Autodesk Inventor part; units mm, degrees
ref_plane "YZ Plane" through (0, 0, 0) normal (1, 0, 0) x (0, 1, 0)
ref_plane "XZ Plane" through (0, 0, 0) normal (0, 1, 0) x (-1, 0, 0)
ref_plane "XY Plane" through (0, 0, 0) normal (0, 0, 1) x (1, 0, 0)
sketch "スケッチ1" plane through (0, 0, 0) normal (0, 0, 1) x (1, 0, 0)
  circle A0 centre (0, 0) radius 4.25
  circle A1 centre (0, 0) radius 4.5
  circle A2 centre (0, 0) radius 5
  line L0 (0, -5) -> (0, -6)
  line L1 (0, -6) -> (8.75, -6)
  line L2 (8.75, -6) -> (-8.75, -6)
  line L3 (0, -6) -> (11.25, -6)
  line L4 (11.25, -6) -> (-11.25, -6)
  line L5 (-11.25, -6) -> (-11.25, -4)
  line L6 (-11.25, -4) -> (11.25, -4)
  line L7 (11.25, -4) -> (11.25, -6)
  circle A3 centre (0, 0) radius 6
  line L8 (-6, 0) -> (-6, -4)
  line L9 (6, 0) -> (6, -4)
  circle A4 centre (0, 0) radius 7.2111
  line L10 (0, 0) -> (0, -3)
  line L11 (0, -3) -> (0, 7.2111)
  line L12 (0, -3) -> (0.75, -3)
  line L13 (0.75, -3) -> (-0.75, -3)
  line L14 (-0.75, -3) -> (-0.75, 5.9529)
  line L15 (0.75, -3) -> (0.75, 5.9529)
  point P0 (4.4721, -4)
  point P1 (-4.4721, -4)
  point P2 (4, -6)
  point P3 (-4, -6)
  point P4 (-0.75, 4.4371)
  point P5 (0.75, 4.4371)
  dimension "d2" = 10
  dimension "d0" = 8.5
  dimension "d1" = 9
  dimension "d3" = 1
  dimension "d4" = 8.75
  dimension "d5" = 17.5
  dimension "d6" = 11.25
  dimension "d7" = 22.5
  dimension "d8" = 2
  dimension "d9" = 12
  dimension "d18" = 3
  dimension "d19" = 0.75
  dimension "d20" = 1.5
extrude "押し出し1" add sketch "スケッチ1" along normal blind 5 contours L6 A1 A0 | A0 L6 | L6 A2 A1 | L6 A3 L0 A2 | A2 L0 A3 L6 | L6 A4 L1 A3 | A3 L2 A4 L6 | L6 L7 L3 L1 A4 | A4 L2 L4 L5 L6
extrude "押し出し2" add sketch "スケッチ1" along normal blind 3 contours A0 L6 L14 L13 L12 L15 | A0 L15 A1 L6 | L15 L12 L10 L11 A0 | A0 L11 A1 L15 | L6 A1 A0 | A0 L6 | L11 L10 L13 L14 A0 | A0 L14 A1 L11 | L15 A2 L6 A1 | A1 L11 A2 L15 | L6 A1 L14 A0 | L6 A2 A1 | A1 L14 A2 L11 | L15 A3 L6 A2 | A2 L11 A3 L15 | L6 A2 L14 A1 | L6 A3 L0 A2 | A2 L14 A3 L11 | L6 A3 L14 A2 | A2 L0 A3 L6 | A3 L9 L6 | L6 L8 A3
extrude "押し出し3" add sketch "スケッチ1" against normal blind 21 contours L15 A2 L6 A1 | A1 L11 A2 L15 | L6 A2 A1 | A1 L14 A2 L11 | L15 A3 L6 A2 | A2 L11 A3 L15 | L6 A2 L14 A1 | L6 A3 L0 A2 | A2 L14 A3 L11 | L6 A3 L14 A2 | A2 L0 A3 L6 | A3 L9 L6 | L6 A4 L1 A3 | A3 L2 A4 L6 | L6 L8 A3
extrude "押し出し4" cut sketch "スケッチ1" along normal blind 1.5 contours A0 L6 L14 L13 L12 L15 | A0 L15 A1 L6 | L15 L12 L10 L11 A0 | A0 L11 A1 L15 | L6 A1 A0 | A0 L6 | L11 L10 L13 L14 A0 | A0 L14 A1 L11 | L6 A1 L14 A0
extrude "押し出し5" cut sketch "スケッチ1" along normal blind 3 contours L15 L12 L10 L11 A0 | A0 L11 A1 L15 | L11 L10 L13 L14 A0 | A0 L14 A1 L11 | A1 L11 A2 L15 | A1 L14 A2 L11 | A2 L11 A3 L15 | A2 L14 A3 L11
extrude "押し出し6" cut sketch "スケッチ1" against normal blind 21 contours A1 L11 A2 L15 | A1 L14 A2 L11 | A2 L11 A3 L15 | A2 L14 A3 L11
sketch "スケッチ2" plane through (-11.25, -4, 5) normal (0, 1, 0) x (1, 0, 0)
  line L0 (22.5, 0) -> (0, 0)
  line L1 (0, 0) -> (0, 2.5)
  line L2 (0, 5) -> (0, 0)
  line L3 (0, 2.5) -> (22.5, 2.5)
  line L4 (22.5, 5) -> (22.5, 0)
  line L5 (22.5, 2.5) -> (20, 2.5)
  line L6 (20, 2.5) -> (2.5, 2.5)
  point P0 (11.25, 5)
  dimension "d25" = 2.5
  dimension "d26" = 17.5
hole "穴1" at (-8.75, -4, 2.5) at (8.75, -4, 2.5) direction (0, -1, 0) diameter 2 end through all
fillet "フィレット1" radius 2 2 edges at (-11.25, -5, 0) (11.25, -5, 0)
properties part number "motor cover1"
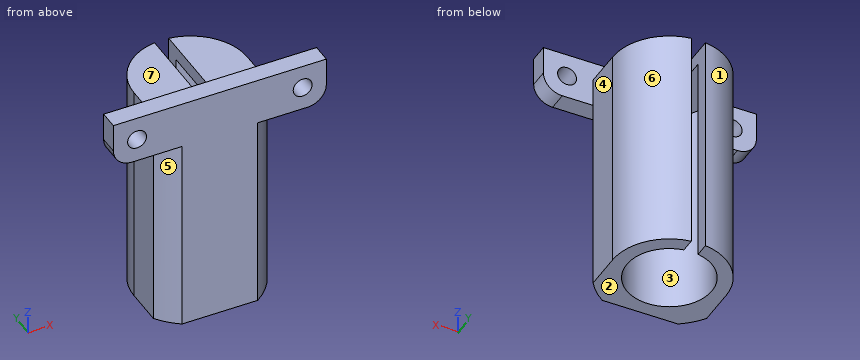
For this review, take the finished solid that the model builds, in its own axes (mm). Face numbers are marked on the shaded views. A direction names the side the tool comes from. Round coordinates to 2 decimals unless told otherwise and drop trailing zeros. Loops run counter-clockwise (first coordinate to the right, second up) from the corner with the lowest first, then second, coordinate; pieces in that order, holes last. Notation, with made-up numbers: (16, 41) - (23, 41) arc R18 ccw to (23, 45) - close; hole circle Ø9 at (57, -17). An arc over 180 degrees is marked (long way). Put each result on its own line as item: value. Start each with the question number.
1. Consider section D-D on z = -4.5. State the section outline as (x, y) points, plus the area to 3 significant figures.
2. Consider section C-C on y = 5. State the section outline as (x, z) points, plus the area to 3 significant figures.
3. Mouldability with a two-part tool opening along X and no side actions: class the marked faces 1, 2, 3 and 4 as +X half, -X half, draft (parallel to the pull), parting line (faces both ways), or undercut.
4. For the marked faces 5, 6 and 7, list the 3-axis set-ups (+Z, -Z, +X, -X, +Y, -Y) from which the entire face can be reached by the end or side of a thin tool; tool diameter is ignored.
5. Consider section B-B on z = 2.5. State the section outline as (x, y) points, plus the area to 3 significant figures.
6. For probe 1 along X at (y, z) = (-0.25, -18); probe 2 along X at (y, z) = (-5.5, 2.5); probe 3 along Z at (x, y) = (-8.75, -4.85), list the stretches that pass through material, from the lowest coordinate up. Write a range as [from, to].
7. Consider section A-A on x = -8.75. State the section outline as (y, z) points.
8. Insertion check: P1, Ø2, axis at x = -6.5, z = -6, coming from the +Y side; P2, Ø1, axis at x = 7, y = -5.5, coming from the -Z side; P3, Ø5, axis at y = -2.5, z = -15, coming from the -X side. Each pin has a flat end and moves straight along its axis. Give the tip position at first contact, or say it passes through.
Result sheet:
1. outline: (-6, -4) arc R7.21 ccw to (-4, -6) - (4, -6) arc R7.21 ccw to (6, -4) - (6, 0) arc R6 ccw to (0.75, 5.95) - (0.75, 4.44) arc R4.5 cw (long way) to (-0.75, 4.44) - (-0.75, 5.95) arc R6 ccw to (-6, 0) - close
1. area: 59.2 mm^2
2. outline: (-3.32, -21) - (-0.75, -21) - (-0.75, 3) - (-3.32, 3) - close; (0.75, -21) - (3.32, -21) - (3.32, 3) - (0.75, 3) - close
2. area: 123 mm^2
3. face 1: -X half
3. face 2: draft
3. face 3: undercut
3. face 4: +X half
4. face 5: -Z, -X, -Y
4. face 6: +Z, -Z, +X, +Y
4. face 7: +Z, +X, -X, +Y
5. outline: (-11.25, -6) - (-9.75, -6) - (-9.75, -4) - (-11.25, -4) - close; (-7.75, -6) - (7.75, -6) - (7.75, -4) - (6, -4) - (6, 0) arc R6 ccw to (0.75, 5.95) - (0.75, -3) - (-0.75, -3) - (-0.75, 5.95) arc R6 ccw to (-6, 0) - (-6, -4) - (-7.75, -4) - close; (9.75, -6) - (11.25, -6) - (11.25, -4) - (9.75, -4) - close
5. area: 128 mm^2
6. probe 1: [-6, -4.49], [4.49, 6]
6. probe 2: [-11.25, -9.75], [-7.75, 7.75], [9.75, 11.25]
6. probe 3: [0, 1.5], [3.5, 5]
7. outline: (-6, 0) - (-4, 0) - (-4, 1.5) - (-6, 1.5) - close; (-6, 3.5) - (-4, 3.5) - (-4, 5) - (-6, 5) - close
8. P1: y = 2.4
8. P2: z = 0
8. P3: x = -6
